The figure shows three views and two pictorial views of one solid part (mm, origin at its lowest corner). Answer the questions. A direction names the side the tool comes from. Give positions to 0.01 mm unless a question says otherwise; leave off trailing zeros. Loops run counter-clockwise (first coordinate to the right, second up) from the corner with the lowest first, then second, coordinate; pieces in that order, holes last. Notation, with made-up numbers: (-36, -2.5) - (-28, -2.5) arc R26 cw to (-28, 19.5) - close; hole circle Ø1 at (48, 80). An arc over 180 degrees is marked (long way). Write item = value, one per line.
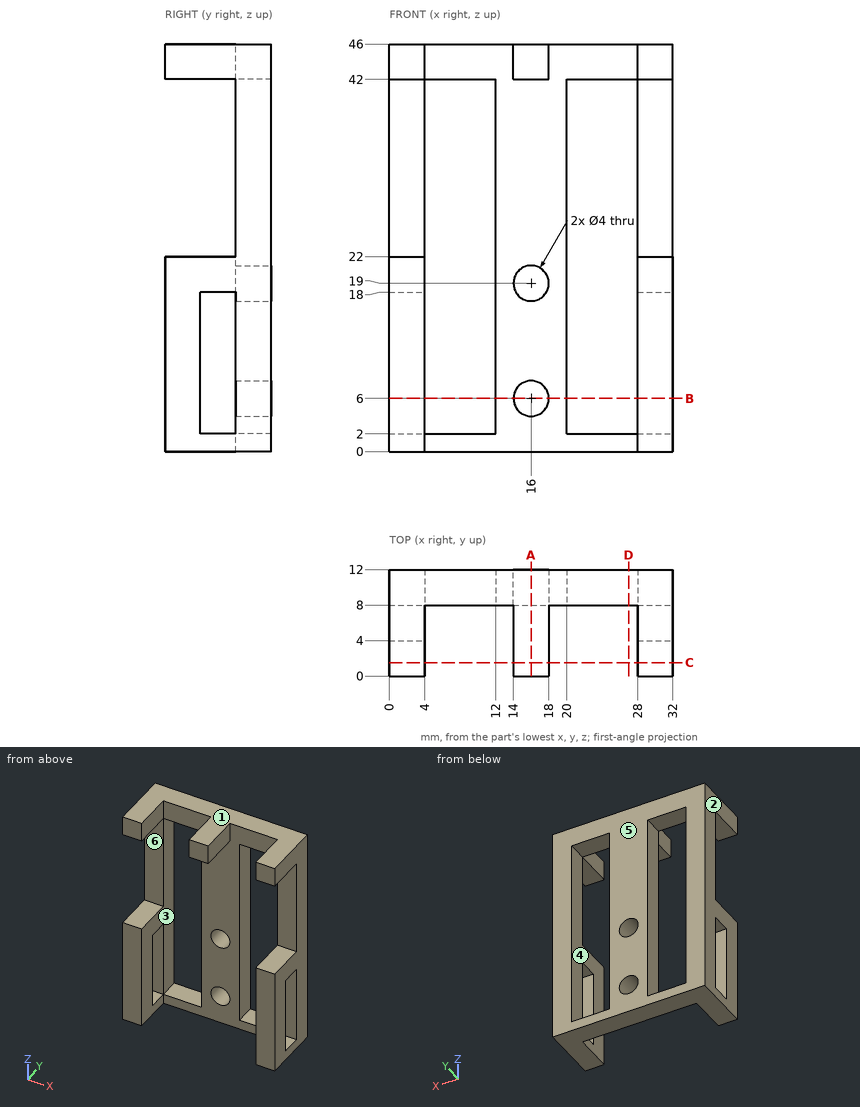
1) Find the intervals of material crossed by probe 1 along Z at (x, y) = (16, 10.3); probe 2 along X at (y, z) = (10.75, 22); probe 3 along X at (y, z) = (2, 16), in increasing order.
Output:
probe_1 = 0 to 4, 8 to 17, 21 to 46
probe_2 = 0 to 4, 12 to 20, 28 to 32
probe_3 = 0 to 4, 28 to 32
2) A cutting plane is placed at D-D on x = 27. Determine the outline of the cut face in (y, z).
Output:
outline = (8, 0) - (12, 0) - (12, 2) - (8, 2) - close; (8, 42) - (12, 42) - (12, 46) - (8, 46) - close
3) A cutting plane is placed at B-B on z = 6. Determine the outline of the cut face in (x, y).
Output:
outline = (0, 0) - (4, 0) - (4, 4) - (0, 4) - close; (0, 8) - (4, 8) - (4, 12) - (0, 12) - close; (12, 8) - (14, 8) - (14, 12) - (12, 12) - close; (18, 8) - (20, 8) - (20, 12) - (18, 12) - close; (28, 0) - (32, 0) - (32, 4) - (28, 4) - close; (28, 8) - (32, 8) - (32, 12) - (28, 12) - close
4) The mould has two halves that part along Z. Classify the marked faces 1, 2, 3 and 4: pulls with the +Z half, pulls with the -Z half, needs draft (parallel to the pull), parting line crosses it, or undercut.
Output:
face_1 = pulls with the +Z half
face_2 = needs draft
face_3 = undercut
face_4 = undercut
5) A tool of negligible diameter and unlimited length cuts with its end or side. For the marked faces 5 and 6, from which of +Z, -Z, +X, -X, +Y, -Y can it reach the whole face along a straight path? Write none if from no direction.
Output:
face_5 = +Z, -Z, +X, -X, +Y
face_6 = +X, -X, -Y
6) This flat-tipped pin is pushed along its axis until it touches: P1, Ø3, axis at x = 30.5, z = 30, coming from the -Y side. Where does it stop, or does it pass through?
Output:
P1 = 8
7) A cutting plane is placed at C-C on y = 1.5. Determine the outline of the cut face in (x, z), then the cut area to 3 significant figures.
Output:
outline = (0, 0) - (4, 0) - (4, 22) - (0, 22) - close; (0, 42) - (4, 42) - (4, 46) - (0, 46) - close; (14, 42) - (18, 42) - (18, 46) - (14, 46) - close; (28, 0) - (32, 0) - (32, 22) - (28, 22) - close; (28, 42) - (32, 42) - (32, 46) - (28, 46) - close
area = 224 mm²
8) A cutting plane is placed at A-A on x = 16. Determine the outline of the cut face in (y, z), then the cut area to 3 significant figures.
Output:
outline = (0, 42) - (8, 42) - (8, 21) - (12, 21) - (12, 46) - (0, 46) - close; (8, 0) - (12, 0) - (12, 4) - (8, 4) - close; (8, 8) - (12, 8) - (12, 17) - (8, 17) - close
area = 184 mm²
